Could you check a few things on this model? Use its own coordinates, in mm. Face numbers are marked on the shaded views. A direction names the side the tool comes from. Coordinates: 2 decimals unless noted, no trailing zeros. Order: outer loops, then holes, each group sorted by start corner. A loop starts at its lowest first (then second) coordinate and runs counter-clockwise, first axis right, second up. Notation, with made-up numbers: (24, 32.25) - (77, 32.25) arc R9 cw to (77, 39.25) - close; hole circle Ø6 at (39, 52.5). An arc over 180 degrees is marked (long way). Answer as a JSON object with one key per item and string values. Group by question number.
(1) Which directions (+Z, -Z, +X, -X, +Y, -Y) give clear straight access to the entire face, cutting with the end or side of a thin tool? Please do the marked faces 1 and 2.
(2) Will these pins go through, and if not, where does the flat tip stop? P1, Ø1, axis at x = 21.5, y = 2, coming from the -Z side; P2, Ø1.5, axis at y = 2.5, z = -43.5, coming from the +X side; P3, Ø5, axis at x = 20, z = 0, coming from the -Y side; P4, Ø2.5, axis at x = 39, y = 3, coming from the -Z side.
(3) Imagine slicing it at B-B, the plane x = 0. Write out the boundary of the cut face in (y, z), and give its area (3 significant figures).
(4) Please list where these lines run through material, in increasing order: probe 1 along Z at (x, y) = (0, 3.25); probe 2 along X at (y, z) = (3.45, 0); probe 3 along Z at (x, y) = (47, 4.8).
(5) Imagine slicing it at D-D, the plane x = 40. Write out the boundary of the cut face in (y, z).
(6) Imagine slicing it at A-A, the plane z = -20. Write out the boundary of the cut face in (x, y).
(7) Imagine slicing it at C-C, the plane y = 1.8. Write out the boundary of the cut face in (x, z), and give its area (3 significant figures).
from build123d import *

# Parameters (mm, degrees)
SKETCH1_W           = 40
SKETCH1_H           = 20
SKETCH1_R           = 2
SKETCH1_W_2         = 20
SKETCH1_H_2         = 40
BOSS_EXTRUDE1_DEPTH = 5
FILLET1_R           = 2
BOSS_EXTRUDE2_DEPTH = 5
FILLET2_R           = 2


with BuildPart() as part:
    # Sketch1 → Boss-Extrude1 (new body)
    with BuildSketch(Plane(origin=(0, 0, 0), x_dir=(1, 0, 0), z_dir=(0, 1, 0))):
        with Locations((30, 0)):
            Rectangle(SKETCH1_W, SKETCH1_H)
        with Locations((20, 0)):
            Circle(SKETCH1_R, mode=Mode.SUBTRACT)
        with Locations((40, 0)):
            Circle(SKETCH1_R, mode=Mode.SUBTRACT)
        Rectangle(SKETCH1_W_2, SKETCH1_H)
        Circle(SKETCH1_R, mode=Mode.SUBTRACT)
        with Locations((0, 30)):
            Rectangle(SKETCH1_W_2, SKETCH1_H_2)
        with Locations((0, 20)):
            Circle(SKETCH1_R, mode=Mode.SUBTRACT)
        with Locations((0, 40)):
            Circle(SKETCH1_R, mode=Mode.SUBTRACT)
    extrude(amount=BOSS_EXTRUDE1_DEPTH)

    # Fillet1
    fillet1_edges = [part.edges().sort_by_distance(p)[0] for p in [
        (-10, 2.5, 10),
        (-10, 2.5, -50),
        (10, 2.5, -50),
        (10, 2.5, -10),
        (50, 2.5, -10),
        (50, 2.5, 10),
    ]]
    fillet(fillet1_edges, radius=FILLET1_R)

    # Sketch2 → Boss-Extrude2 (add)
    with BuildSketch(Plane(origin=(0, 5, 0), x_dir=(1, 0, 0), z_dir=(0, 1, 0))):
        Polygon((10, 30), (30, 10), (7.050252532, 7.050252532), align=None)
    extrude(amount=-BOSS_EXTRUDE2_DEPTH)

    # Fillet2
    fillet2_edges = [part.edges().sort_by_distance(p)[0] for p in [
        (10, 2.5, -30),
        (30, 2.5, -10),
    ]]
    fillet(fillet2_edges, radius=FILLET2_R)


solid = part.part
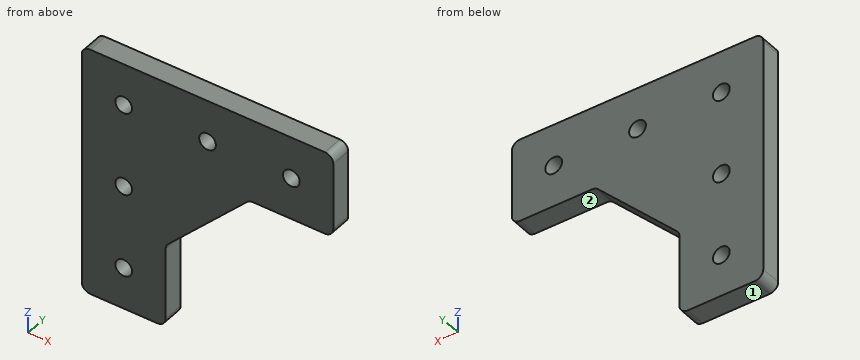
Result set:
{
 "1": {"face 1": "-Z, +X, -X, +Y, -Y", "face 2": "-Z, +X, +Y, -Y"},
 "2": {"P1": "stops at z = -19", "P2": "stops at x = 10", "P3": "stops at y = 0", "P4": "stops at z = -10"},
 "3": {"outline": "(0, -50) - (5, -50) - (5, -42) - (0, -42) - close; (0, -38) - (5, -38) - (5, -22) - (0, -22) - close; (0, -18) - (5, -18) - (5, -2) - (0, -2) - close; (0, 2) - (5, 2) - (5, 10) - (0, 10) - close", "area": "240 mm^2"},
 "4": {"probe 1": "z = -50 to -42, -38 to -22, -18 to -2, 2 to 10", "probe 2": "x = -10 to -2, 2 to 18, 22 to 38, 42 to 50", "probe 3": "z = -10 to 10"},
 "5": {"outline": "(0, -10) - (5, -10) - (5, -2) - (0, -2) - close; (0, 2) - (5, 2) - (5, 10) - (0, 10) - close"},
 "6": {"outline": "(-10, 0) - (-2, 0) - (-2, 5) - (-10, 5) - close; (2, 0) - (20, 0) - (20, 5) - (2, 5) - close"},
 "7": {"outline": "(-10, -48) arc R2 ccw to (-8, -50) - (8, -50) arc R2 ccw to (10, -48) - (10, -30.83) arc R2 cw to (10.59, -29.41) - (29.41, -10.59) arc R2 cw to (30.83, -10) - (48, -10) arc R2 ccw to (50, -8) - (50, 8) arc R2 ccw to (48, 10) - (-8, 10) arc R2 ccw to (-10, 8) - close; hole circle Ø4 at (0, -40); hole circle Ø4 at (0, -20); hole circle Ø4 at (0, 0); hole circle Ø4 at (20, 0); hole circle Ø4 at (40, 0)", "area": "2,130 mm^2"}
}
